For this review, use the dimensioned drawing (mm, ordinates from the lowest corner) and the shaded views. Round coordinates to 2 decimals unless told otherwise and drop trailing zeros. Write each loop counter-clockwise with the first axis right and the second up, starting at its lowest first coordinate (ties: lowest second). Pieces come first, ordered by that corner, then holes. Notation, with made-up numbers: M 49.5,78 L 100.5,78 A28 ccw 100.5,110 Z; hole C -36,-24 d9. An arc over 180 degrees is marked long. One line per question, with ' | ' between items. Start each with the question number.
Item 1: Add section B-B, the plane x = 38.1. State the section outline as (y, z) points (1 decimal).
Item 2: For L1, parallel to X at y = 3.25, z = 63.5; L2, parallel to X at y = 4.45, z = 61; L3, parallel to X at y = 1.2, z = 40.5, list the stretches that pass through material, from the lowest coordinate up.
Item 3: Add section C-C, the plane x = 12.7. State the section outline as (y, z) points (1 decimal).
Item 4: Add section D-D, the plane y = 2.65. State the section outline as (x, z) points, and give its area (3 significant figures).
Item 5: Insertion check: pin 1 Ø2 at (x, y) = (37, 3) entering from -Z. The pin has a flat end and moves straight along its axis. Give the tip position at first contact, or say it passes through.
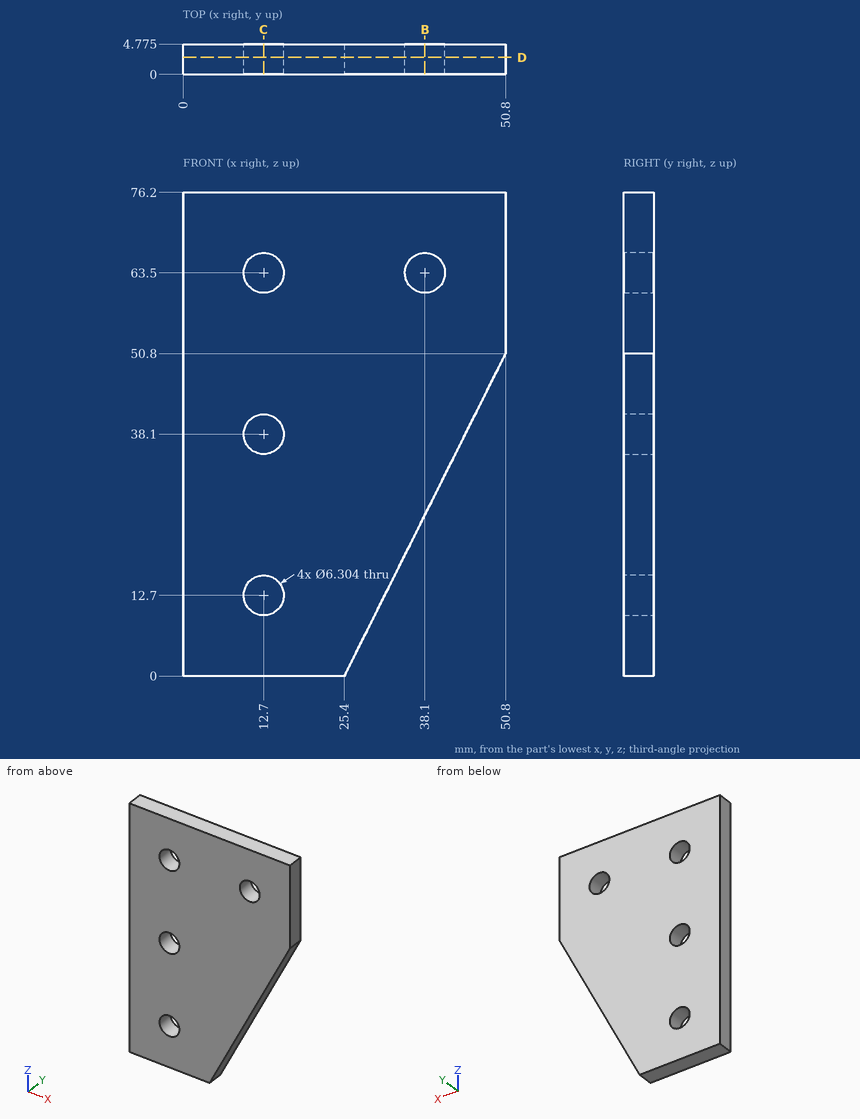
Computed values:
1) outline: M 0,25.4 L 4.8,25.4 L 4.8,60.3 L 0,60.3 Z; M 0,66.7 L 4.8,66.7 L 4.8,76.2 L 0,76.2 Z
2) L1: x = 0 to 9.55, 15.85 to 34.95, 41.25 to 50.8 | L2: x = 0 to 10.78, 14.62 to 36.18, 40.02 to 50.8 | L3: x = 0 to 10.66, 14.74 to 45.65
3) outline: M 0,0 L 4.8,0 L 4.8,9.5 L 0,9.5 Z; M 0,15.9 L 4.8,15.9 L 4.8,34.9 L 0,34.9 Z; M 0,41.3 L 4.8,41.3 L 4.8,60.3 L 0,60.3 Z; M 0,66.7 L 4.8,66.7 L 4.8,76.2 L 0,76.2 Z
4) outline: M 0,0 L 25.4,0 L 50.8,50.8 L 50.8,76.2 L 0,76.2 Z; hole C 12.7,12.7 d6.3; hole C 12.7,38.1 d6.3; hole C 12.7,63.5 d6.3; hole C 38.1,63.5 d6.3 | area: 3,100 mm^2
5) pin 1: stops at z = 21.2
